```python
from build123d import *

# Parameters (mm, degrees)
SKETCH1_W               = 38
SKETCH1_H               = 44
SKETCH1_R               = 2
BOSS_EXTRUDE1_DEPTH     = 10
SKETCH2_R               = 7
BOSS_EXTRUDE2_DEPTH     = 13
FILLET1_R               = 3
FILLET2_R               = 7
CUT_EXTRUDE1_DEPTH      = 42.060930335
CUT_EXTRUDE1_DEPTH_BACK = 42.060930335
SKETCH3_W               = 24
SKETCH3_H               = 30
BOSS_EXTRUDE3_START     = 8
SKETCH4_R               = 7
BOSS_EXTRUDE3_DEPTH     = 8
CUT_EXTRUDE2_DEPTH      = 42.060930335
CUT_EXTRUDE2_DEPTH_BACK = 42.060930335
SKETCH8_R               = 5
CUT_EXTRUDE3_DEPTH      = 50.859803449
CUT_EXTRUDE3_DEPTH_BACK = 13
SKETCH9_R               = 1.75
FILLET3_SIZE            = 4
FILLET3_SIZE_2          = 1


# Some blends are built 0.0001 mm under size
with BuildPart() as part:
    # Sketch1 → Boss-Extrude1 (new, symmetric)
    with BuildSketch(Plane.XY):
        Rectangle(SKETCH1_W, SKETCH1_H)
        with Locations((-15, 16)):
            Circle(SKETCH1_R, mode=Mode.SUBTRACT)
        with Locations((15, 16)):
            Circle(SKETCH1_R, mode=Mode.SUBTRACT)
        with Locations((15, -16)):
            Circle(SKETCH1_R, mode=Mode.SUBTRACT)
        with Locations((-15, -16)):
            Circle(SKETCH1_R, mode=Mode.SUBTRACT)
    extrude(amount=BOSS_EXTRUDE1_DEPTH, both=True)

    # Sketch2 → Boss-Extrude2 (add)
    with BuildSketch(Plane(origin=(0, 22, 0), x_dir=(1, 0, 0), z_dir=(0, 1, 0))):
        with Locations(Location((0, 0, 0), (0, 0, 90))):
            Circle(SKETCH2_R)
    extrude(amount=BOSS_EXTRUDE2_DEPTH)

    # Fillet1
    fillet1_edges = [part.edges().sort_by_distance(p)[0] for p in [
        (0, 22, 7),
    ]]
    fillet(fillet1_edges, radius=FILLET1_R - 0.0001)  # a hair under: the kernel refuses the full size

    # Fillet2
    fillet2_edges = [part.edges().sort_by_distance(p)[0] for p in [
        (0, 35, 7),
    ]]
    fillet(fillet2_edges, radius=FILLET2_R)

    # Sketch3 → Cut-Extrude1 (cut, two sides: drawn at the far end of the back side and taken through both)
    with BuildSketch(Plane.XY.offset(-CUT_EXTRUDE1_DEPTH_BACK)):
        Rectangle(SKETCH3_W, SKETCH3_H)
    extrude(amount=CUT_EXTRUDE1_DEPTH + CUT_EXTRUDE1_DEPTH_BACK, mode=Mode.SUBTRACT)

    # Sketch4 → Boss-Extrude3 (add)
    with BuildSketch(Plane.XZ.offset(22).offset(BOSS_EXTRUDE3_START)):
        with Locations(Location((0, 0, 0), (0, 0, 270))):
            Circle(SKETCH4_R)
    extrude(amount=-BOSS_EXTRUDE3_DEPTH)

    # Sketch7 → Cut-Revolve1 (revolve, cut)
    with BuildSketch(Plane(origin=(0, 0, 0), x_dir=(0, 0, -1), z_dir=(1, 0, 0)), mode=Mode.PRIVATE) as cut_revolve1_sk:
        Polygon((0, -30), (0, -12.56), (2.5, -12.56), (2.5, -18), (5, -18), (5, -30), align=None)
    revolve(cut_revolve1_sk.sketch.rotate(Axis((0, -30, 0), (0, -1, 0)), 180), axis=Axis((0, -30, 0), (0, -1, 0)), mode=Mode.SUBTRACT)

    # Sketch8 → Cut-Extrude2 (cut, two sides: drawn at the far end of the back side and taken through both)
    with BuildSketch(Plane(origin=(0, 0, 0), x_dir=(0, 0, -1), z_dir=(1, 0, 0)).offset(-CUT_EXTRUDE2_DEPTH_BACK)):
        Circle(SKETCH8_R)
    extrude(amount=CUT_EXTRUDE2_DEPTH + CUT_EXTRUDE2_DEPTH_BACK, mode=Mode.SUBTRACT)

    # Sketch9 → Cut-Extrude3 (cut, two sides: drawn at the far end of the back side and taken through both)
    with BuildSketch(Plane.XZ.offset(-15).offset(-CUT_EXTRUDE3_DEPTH_BACK)):
        with Locations(Location((0, 0, 0), (0, 0, 90))):
            Circle(SKETCH9_R)
    extrude(amount=CUT_EXTRUDE3_DEPTH + CUT_EXTRUDE3_DEPTH_BACK, mode=Mode.SUBTRACT)

    # Fillet3
    # an asymmetric fillet: 4, 1 mm, written as the material it adds along each edge
    with BuildSketch(Plane(origin=(12, -15, -10), x_dir=(0, 1, 0), z_dir=(0, 0, 1))) as fillet3_piece_1:
        with BuildLine():
            Bezier((FILLET3_SIZE, 0), (0, 0), (0, FILLET3_SIZE_2), weights=[1, 0.707106781, 1])
            Line((0, FILLET3_SIZE_2), (0, 0))
            Line((0, 0), (FILLET3_SIZE, 0))
        make_face()
    extrude(amount=20)
    with BuildSketch(Plane(origin=(12, 15, -10), x_dir=(0, -1, 0), z_dir=(0, 0, 1))) as fillet3_piece_2:
        with BuildLine():
            Bezier((FILLET3_SIZE_2, 0), (0, 0), (0, -FILLET3_SIZE), weights=[1, 0.707106781, 1])
            Line((0, -FILLET3_SIZE), (0, 0))
            Line((0, 0), (FILLET3_SIZE_2, 0))
        make_face()
    extrude(amount=20)
    with BuildSketch(Plane(origin=(-12, -15, 10), x_dir=(0, 1, 0), z_dir=(0, 0, -1)), Plane(origin=(-12, 15, 10), x_dir=(1, 0, 0), z_dir=(0, 0, -1))) as fillet3_piece_3:
        with BuildLine():
            Bezier((FILLET3_SIZE_2, 0), (0, 0), (0, FILLET3_SIZE), weights=[1, 0.707106781, 1])
            Line((0, FILLET3_SIZE), (0, 0))
            Line((0, 0), (FILLET3_SIZE_2, 0))
        make_face()
    extrude(amount=20)


solid = part.part
```
For this review, take the finished solid that the model builds, in its own axes (mm). A direction names the side the tool comes from. Give positions to 0.01 mm unless a question says otherwise; leave off trailing zeros. Write each loop counter-clockwise with the first axis right and the second up, starting at its lowest first coordinate (ties: lowest second). Pieces come first, ordered by that corner, then holes. Notation, with made-up numbers: M 9,49 L 29,49 A17 cw 29,81 Z; hole C 40.5,37 d8. An arc over 180 degrees is marked long. Answer as a JSON object with one key per item and string values. Group by question number.
Item 1: Tool access review of faces 5 (the flat face through (-4, 15, 0)), 6 (the flat face through (13, 0, -10)), 7 (the cylindrical face through (0, -24, -5)): name each direction out of +Z, -Z, +X, -X, +Y, -Y from which nothing blocks a thin tool from reaching the whole face with its end or side.
Item 2: Draft analysis for pull direction X (two halves, no side actions). For faces 1 (the flat face through (19, -5.2, 0.1)), 2 (the cylindrical face through (15.45, -4.88, 1.08)), 3 (the flat face through (0, 28, 0)), 4 (the cylindrical face through (6.834, 26.479, 1.517)), state which applies: +X half, -X half, draft (parallel to the pull), parting line (faces both ways), or undercut.
Item 3: For probe 1 along X at (y, z) = (20.75, 0); probe 2 along Y at (x, z) = (-15, -6.25); probe 3 along Y at (x, z) = (-13.5, 0.5), list the stretches that pass through material, from the lowest coordinate up. Write a range as [from, to].
Item 4: For pin 1 Ø4.5 at (x, z) = (0, 0) entering from -Y; pin 2 Ø8 at (x, z) = (0, 0) entering from -Y; pin 3 Ø1 at (x, z) = (-9.5, -5) entering from +Y, all flat-tipped, find the tip position at first contact; note any pin that passes through.
Item 5: Consider section B-B on y = 16. Write out the cut boundary in (x, z).
Item 6: Consider section A-A on x = -15. Write out the cut boundary in (y, z), plus the area to 3 significant figures.
Item 7: Consider section C-C on y = 8. Write out the cut boundary in (x, z).
Item 8: Consider section D-D on x = 0. Count the separate pieces of the cut face and the enclosed holes in it, plus the area to 3 significant figures.
Check result:
{
 "1": {"face 5": "+Z, -Z", "face 6": "-Z, +X, -X, +Y, -Y", "face 7": "-Y"},
 "2": {"face 1": "+X half", "face 2": "draft", "face 3": "undercut", "face 4": "parting line"},
 "3": {"probe 1": "x = [-19, -1.75], [1.75, 19]", "probe 2": "y = [-22, -18], [-14, 14], [18, 22]", "probe 3": "y = [-22, -17.32], [-14.68, -4.97], [4.97, 14.68], [17.32, 22]"},
 "4": {"pin 1": "stops at y = 15", "pin 2": "stops at y = -18", "pin 3": "stops at y = 22"},
 "5": {"outline": "M -19,-10 L -17,-10 L -17,10 L -19,10 Z; M -13,-10 L 13,-10 L 13,10 L -13,10 Z; M 17,-10 L 19,-10 L 19,10 L 17,10 Z; hole C 0,0 d3.5"},
 "6": {"outline": "M -22,-10 L -18,-10 L -18,10 L -22,10 Z; M -14,-10 L 14,-10 L 14,10 L -14,10 Z; M 18,-10 L 22,-10 L 22,10 L 18,10 Z; hole C 0,0 d10", "area": "641 mm^2"},
 "7": {"outline": "M -19,-10 L -12,-10 L -12,10 L -19,10 Z; M 12,-10 L 19,-10 L 19,10 L 12,10 Z"},
 "8": {"separate pieces": "3", "enclosed holes": "0", "area": "376 mm^2"}
}
